Verification items for the finished model (mm, model axes). A direction names the side the tool comes from. Give positions to 0.01 mm unless a question says otherwise; leave off trailing zeros. Write each loop counter-clockwise with the first axis right and the second up, starting at its lowest first coordinate (ties: lowest second). Pieces come first, ordered by that corner, then holes. Notation, with made-up numbers: (81.25, 5.5) - (115.25, 5.5) arc R19 ccw to (115.25, 22.5) - close; hole circle Ø2 at (20.5, -29). An arc over 180 degrees is marked (long way). Answer as a JSON object with one key per item and string values. Group by question number.
Item 1: Draft check along Y on faces 1 (the face through (-98, -30, 0)), 2 (the face through (-110, 0, 13)), 3 (the face through (-164.236, -30, 11)), 4 (the face through (-93, -41.275, 11)). Enter one of: +Y half, -Y half, draft (parallel to the pull), parting line (faces both ways), or undercut.
Item 2: Sectioned sample at D-D, the plane y = -6.5. Record the boundary of the cut face in (x, z).
Item 3: Tool access check on faces 5 (the face through (-185, -18.999, 13)), 6 (the face through (-44.12, -51, 39)), 7 (the face through (-76.962, -51, 11)). Record the directions out of +Z, -Z, +X, -X, +Y, -Y that give a thin tool (end or side, any length) a straight path to the whole face; none if there is none.
Item 4: Go/stop test with flat-tipped pins: pin 1 (15 mm diameter, centred on x = -194.21, z = 22.35, fed in from +Y); pin 2 (6.5 mm diameter, centred on x = -89.5, z = 9.5, fed in from -Y) (3 decimals); pin 3 (18 mm diameter, centred on x = -75, y = -30.5, fed in from +Z); pin 4 (1 mm diameter, centred on x = -153.5, y = -38.5, fed in from -Z). Record where each tip stops, or that it passes through.
Item 5: Sectioned sample at B-B, the plane z = 17.5. Record the boundary of the cut face in (x, y) (3 decimals), and give its area (3 significant figures).
Item 6: Sectioned sample at C-C, the plane x = -199. Record the boundary of the cut face in (y, z) (3 decimals), and give its area (3 significant figures).
Item 7: Scan lines: line 1 along X through (y, z) = (-54, 13); line 2 along X through (y, z) = (-43, 21); line 3 along Y through (x, z) = (-190, 44) (3 decimals). Record each from-to range of solid material in increasing order. Write a range as [from, to].
Item 8: Sectioned sample at A-A, the plane y = -49. Record the boundary of the cut face in (x, z).
```python
from build123d import *

# Parameters (mm, degrees)
F0_R     = 12.7
F1_DEPTH = 60.325
F3_DEPTH = 19.05
F4_DEPTH = 19.05
F5_R     = 6.35
F6_DEPTH = 22.352
F8_R     = 3.302
F7_W     = 69.4968977088
F7_H     = 22.3266
F9_DEPTH = 63.5


with BuildPart() as f1:
    # F0 (on Front) → F1 (new body)
    with BuildSketch(Plane.XZ):
        with BuildLine():
            Line((-194.2084, 0), (-102.362, 0))
            Line((-102.362, 0), (-104.313945544, 7.2784410115))
            ThreePointArc((-104.313945544, 7.2784410115), (-129.5850257878, 8.8118186082), (-150.9776, 22.352))
            Line((-150.9776, 22.352), (-171.8564, 22.352))
            ThreePointArc((-171.8564, 22.352), (-210.0136507731, 38.1572507731), (-194.2084, 0))
        make_face()
        with Locations((-194.2084, 22.352)):
            Circle(F0_R, mode=Mode.SUBTRACT)
        with BuildLine():
            ThreePointArc((-150.9776, 22.352), (-129.5850257878, 8.8118186082), (-104.313945544, 7.2784410115))
            Line((-104.313945544, 7.2784410115), (-108.3564, 22.352))
            Line((-108.3564, 22.352), (-150.9776, 22.352))
        make_face()
        with BuildLine():
            ThreePointArc((-104.313945544, 7.2784410115), (-89.4508847111, 12.6611726116), (-76.962, 22.352))
            Line((-76.962, 22.352), (-108.3564, 22.352))
            Line((-108.3564, 22.352), (-104.313945544, 7.2784410115))
        make_face()
        with BuildLine():
            Line((-102.362, 0), (-76.962, 0))
            Line((-76.962, 0), (-76.962, 22.352))
            ThreePointArc((-76.962, 22.352), (-89.4508847111, 12.6611726116), (-104.313945544, 7.2784410115))
            Line((-104.313945544, 7.2784410115), (-102.362, 0))
        make_face()
        with BuildLine():
            Line((-76.962, 0), (0, 0))
            Line((0, 0), (0, 14.478))
            ThreePointArc((0, 14.478), (-2.3062412049, 20.0457587951), (-7.874, 22.352))
            Line((-7.874, 22.352), (-44.1198, 22.352))
            Line((-44.1198, 22.352), (-76.962, 22.352))
            Line((-76.962, 22.352), (-76.962, 0))
        make_face()
    extrude(amount=F1_DEPTH)

    # F2 (on face) → F3 (join)
    with BuildSketch(Plane.XZ.offset(60.325)):
        with BuildLine():
            ThreePointArc((-63.1698000533, 57.15), (-66.743984667, 38.4343576399), (-76.962, 22.352))
            Line((-76.962, 22.352), (-44.1198, 22.352))
            Line((-44.1198, 22.352), (-44.1198, 52.07))
            ThreePointArc((-44.1198, 52.07), (-45.6076975516, 55.6621024484), (-49.1998, 57.15))
            Line((-49.1998, 57.15), (-63.1698000533, 57.15))
        make_face()
    extrude(amount=-F3_DEPTH)

    # F2 (on face) → F4 (cut)
    with BuildSketch(Plane.XZ.offset(60.325)):
        with BuildLine():
            ThreePointArc((-104.313945544, 7.2784410115), (-89.4508847111, 12.6611726116), (-76.962, 22.352))
            Line((-76.962, 22.352), (-108.3564, 22.352))
            Line((-108.3564, 22.352), (-104.313945544, 7.2784410115))
        make_face()
        with BuildLine():
            Line((-76.962, 0), (-76.962, 22.352))
            ThreePointArc((-76.962, 22.352), (-89.4508847111, 12.6611726116), (-104.313945544, 7.2784410115))
            Line((-104.313945544, 7.2784410115), (-102.362, 0))
            Line((-102.362, 0), (-76.962, 0))
        make_face()
    extrude(amount=-F4_DEPTH, mode=Mode.SUBTRACT)

    # F5 (on face) → F6 (cut, through all)
    with BuildSketch(Plane.XY.offset(22.352)):
        with Locations((-38.862, -22.352)):
            Circle(F5_R)
    extrude(amount=-F6_DEPTH, mode=Mode.SUBTRACT)

    # F8
    f8_edges = [f1.edges().sort_by_distance(p)[0] for p in [
        (-171.8564, -30.1625, 22.352),
        (-44.1198, -50.8, 22.352),
    ]]
    fillet(f8_edges, radius=F8_R)

    # F7 (on face) → F9 (cut, symmetric)
    with BuildSketch(Plane.XY.offset(22.352)):
        with Locations((-198.9848488544, -30.1625)):
            Rectangle(F7_W, F7_H)
    extrude(amount=F9_DEPTH, both=True, mode=Mode.SUBTRACT)


solid = f1.part
```
Geometry check:
{
 "1": {"face 1": "draft", "face 2": "+Y half", "face 3": "undercut", "face 4": "-Y half"},
 "2": {"outline": "(-194.21, 0) - (0, 0) - (0, 14.48) arc R7.87 ccw to (-7.87, 22.35) - (-168.77, 22.35) arc R3.3 cw to (-172.04, 25.23) arc R22.35 ccw (long way) to start; hole circle Ø25.4 at (-194.21, 22.35)"},
 "3": {"face 5": "+Z, -Z, -X", "face 6": "+Z, +X, +Y, -Y", "face 7": "+Z, -Z, -Y"},
 "4": {"pin 1": "through", "pin 2": "y = -41.275", "pin 3": "z = 22.35", "pin 4": "z = 0"},
 "5": {"outline": "(-216.027, -60.325) - (-205.945, -60.325) - (-205.945, -41.326) - (-216.027, -41.326) - close; (-216.027, -18.999) - (-205.945, -18.999) - (-205.945, 0) - (-216.027, 0) - close; (-182.472, -60.325) - (-107.055, -60.325) - (-107.055, -41.275) - (-76.962, -41.275) - (-76.962, -60.325) - (-0.603, -60.325) - (-0.603, 0) - (-182.472, 0) - (-182.472, -18.999) - (-164.236, -18.999) - (-164.236, -41.326) - (-182.472, -41.326) - close; hole circle Ø12.7 at (-38.862, -22.352)", "area": "10,200 mm^2"},
 "6": {"outline": "(-60.325, 0.52) - (-41.326, 0.52) - (-41.326, 10.591) - (-60.325, 10.591) - close; (-60.325, 34.113) - (-41.326, 34.113) - (-41.326, 44.184) - (-60.325, 44.184) - close; (-18.999, 0.52) - (0, 0.52) - (0, 10.591) - (-18.999, 10.591) - close; (-18.999, 34.113) - (0, 34.113) - (0, 44.184) - (-18.999, 44.184) - close", "area": "765 mm^2"},
 "7": {"line 1": "[-214.51, -202.8], [-185.62, -105.85], [-76.96, 0]", "line 2": "[-216.52, -206.84], [-181.58, -107.99], [-76.96, -3.46]", "line 3": "[-60.325, -41.326], [-18.999, 0]"},
 "8": {"outline": "(-194.21, 0) - (-102.36, 0) - (-108.36, 22.35) - (-168.77, 22.35) arc R3.3 cw to (-172.04, 25.23) arc R22.35 ccw (long way) to start; (-76.96, 0) - (0, 0) - (0, 14.48) arc R7.87 ccw to (-7.87, 22.35) - (-40.82, 22.35) arc R3.3 cw to (-44.12, 25.65) - (-44.12, 52.07) arc R5.08 ccw to (-49.2, 57.15) - (-63.17, 57.15) arc R50.8 cw to (-76.96, 22.35) - close; hole circle Ø25.4 at (-194.21, 22.35)"}
}
